```python
from build123d import *

# Parameters (mm, degrees)
BOSS_EXTRUDE1_DEPTH = 12.7
BOSS_EXTRUDE3_DEPTH = 5.08
SKETCH4_R           = 3.175
CUT_EXTRUDE2_DEPTH  = 5.08


with BuildPart() as part:
    # Sketch1 → Boss-Extrude1 (new body)
    with BuildSketch(Plane(origin=(0, 0, 0), x_dir=(1, 0, 0), z_dir=(0, 1, 0))):
        with BuildLine():
            Line((0, 0), (63.5, 0))
            ThreePointArc((63.5, 0), (71.721251762, 11.884057145), (85.741073105, 8.382))
            Line((85.741073105, 8.382), (123.841073105, 8.382))
            Line((123.841073105, 8.382), (123.841073105, 13.462))
            Line((123.841073105, 13.462), (87.814773179, 13.462))
            ThreePointArc((87.814773179, 13.462), (72.969121208, 17.483987595), (60.541247082, 8.422105263))
            ThreePointArc((60.541247082, 8.422105263), (58.206316594, 5.979191272), (54.948835326, 5.08))
            Line((54.948835326, 5.08), (8.551164674, 5.08))
            ThreePointArc((8.551164674, 5.08), (5.293683406, 5.979191272), (2.958752918, 8.422105263))
            ThreePointArc((2.958752918, 8.422105263), (-9.469121208, 17.483987595), (-24.314773179, 13.462))
            Line((-24.314773179, 13.462), (-60.341073105, 13.462))
            Line((-60.341073105, 13.462), (-60.341073105, 8.382))
            Line((-60.341073105, 8.382), (-22.241073105, 8.382))
            ThreePointArc((-22.241073105, 8.382), (-8.221251762, 11.884057145), (0, 0))
        make_face()
    extrude(amount=BOSS_EXTRUDE1_DEPTH)

    # Sketch3 → Boss-Extrude3 (add)
    with BuildSketch(Plane(origin=(0, 0, -13.462), x_dir=(-1, 0, 0), z_dir=(0, 0, -1))):
        Polygon((81.931073105, -16.1036), (60.341073105, -16.1036), (60.341073105, 28.8036), (60.341073105, 42.5196), (81.931073105, 42.5196), (81.931073105, 28.8036), (81.931073105, 21.8059), (66.691073105, 21.8059), (66.691073105, -9.1059), (81.931073105, -9.1059), align=None)
        Polygon((-123.841073105, -16.1036), (-123.841073105, 28.8036), (-123.841073105, 42.5196), (-145.431073105, 42.5196), (-145.431073105, 28.8036), (-145.431073105, 21.8059), (-130.191073105, 21.8059), (-130.191073105, -9.1059), (-145.431073105, -9.1059), (-145.431073105, -16.1036), align=None)
    extrude(amount=-BOSS_EXTRUDE3_DEPTH)

    # Sketch4 → Cut-Extrude2 (cut)
    with BuildSketch(Plane(origin=(0, 0, -13.462), x_dir=(-1, 0, 0), z_dir=(0, 0, -1))):
        with Locations((-140.351073105, 37.32276)):
            Circle(SKETCH4_R)
        with Locations((-128.921073105, 37.32276)):
            Circle(SKETCH4_R)
        with Locations((65.421073105, 37.32276)):
            Circle(SKETCH4_R)
        with Locations((76.851073105, 37.32276)):
            Circle(SKETCH4_R)
    extrude(amount=-CUT_EXTRUDE2_DEPTH, mode=Mode.SUBTRACT)


solid = part.part
```
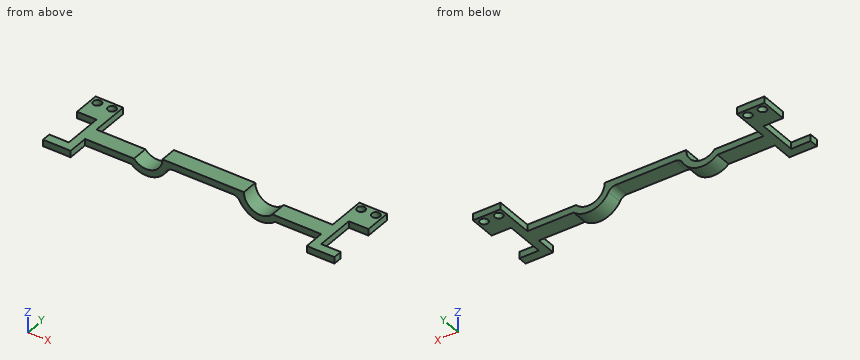
Work out the finished part from the listing and answer in its coordinate system (mm). Give positions to 0.01 mm unless a question says otherwise; leave off trailing zeros. Loops run counter-clockwise (first coordinate to the right, second up) from the corner with the lowest first, then second, coordinate; pieces in that order, holes last. Notation, with made-up numbers: (-22.5, 62) - (27.5, 62) arc R25 cw to (27.5, 99) - close; hole circle Ø9 at (82.5, 74.5). An arc over 180 degrees is marked (long way). Use CSV: the item, a comma, the result in double quotes. Start each with the question number.
(1) Find section A-A, the plane y = 31. Determine the outline of the cut face in (x, z).
(2) Each of these flat-tipped pins is pushed along its axis until it touches: pin 1 (10 mm diameter, centred on x = -65.42, y = 37.32, fed in from +Z); pin 2 (4 mm diameter, centred on y = -6, z = -12, fed in from -X); pin 3 (10 mm diameter, centred on x = -76.85, y = 37.32, fed in from -Z). Where does it stop, or does it pass through?
(3) Find the intervals of material crossed by L1, parallel to X at y = 31, z = -10.5; L2, parallel to X at y = 8.5, z = -10; L3, parallel to Z at x = 125, y = 6, in increasing order.
(4) Find section D-D, the plane x = 53. Determine the outline of the cut face in (y, z), plus the area to 3 significant figures.
(5) Find section B-B, the plane z = -10.75. Count the separate pieces of the cut face and the enclosed holes in it, plus the area to 3 significant figures.
(6) Find section C-C, the plane y = -2. Determine the outline of the cut face in (x, z), plus the area to 3 significant figures.
Results found:
1,outline,"(-81.93, -13.46) - (-60.34, -13.46) - (-60.34, -8.38) - (-81.93, -8.38) - close; (123.84, -13.46) - (145.43, -13.46) - (145.43, -8.38) - (123.84, -8.38) - close"
2,pin 1,"z = -8.38"
2,pin 2,"x = -66.69"
2,pin 3,"z = -13.46"
3,L1,"-81.93 to -60.34, 123.84 to 145.43"
3,L2,"-66.69 to -20.53, -4.87 to 2, 61.5 to 68.37, 84.03 to 130.19"
3,L3,"-13.46 to -8.38"
4,outline,"(0, -5.08) - (12.7, -5.08) - (12.7, 0) - (0, 0) - close"
4,area,"64.5 mm^2"
5,separate pieces,"4"
5,enclosed holes,"4"
5,area,"2,690 mm^2"
6,outline,"(-66.69, -13.46) - (-60.34, -13.46) - (-60.34, -8.38) - (-66.69, -8.38) - close; (123.84, -13.46) - (130.19, -13.46) - (130.19, -8.38) - (123.84, -8.38) - close"
6,area,"64.5 mm^2"
